Drawing for the job (mm, zero at the part's lowest x, y, z). A direction names the side the tool comes from. Give positions to 0.01 mm unless a question says otherwise; leave off trailing zeros. Loops run counter-clockwise (first coordinate to the right, second up) from the corner with the lowest first, then second, coordinate; pieces in that order, holes last. Notation, with made-up numbers: (40, -36) -> (92, -36) arc R23 ccw to (92, -20) -> close; hole circle Ø7 at (-5.5, -22.5). An arc over 180 degrees is marked (long way). Answer in a Markdown table with one row per item. Add a question column.
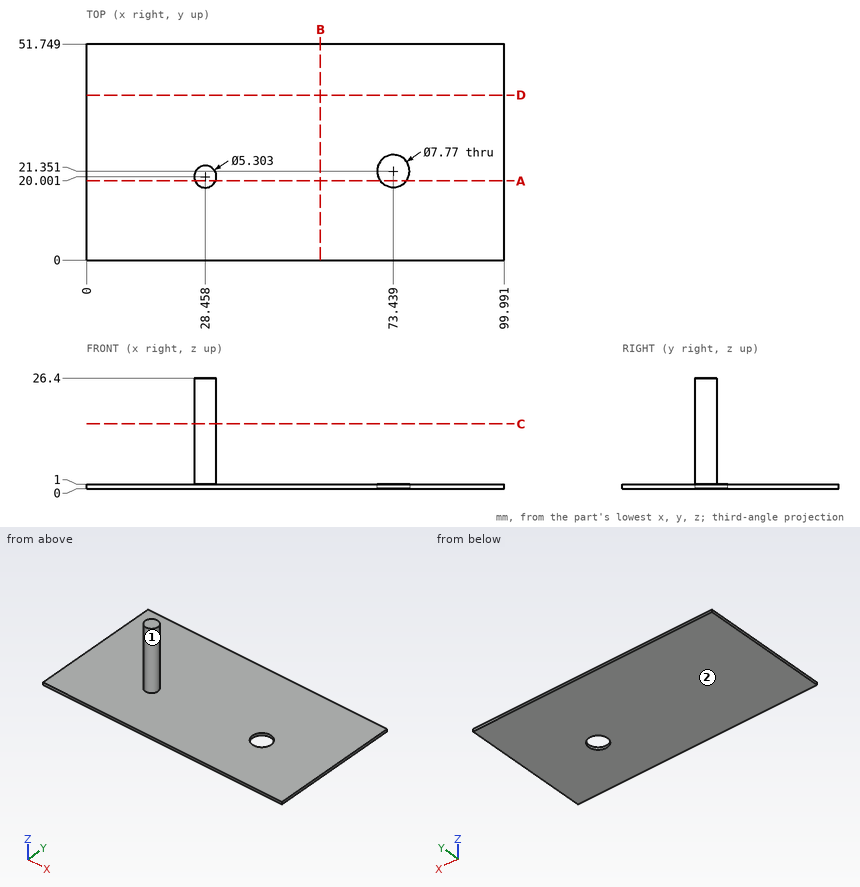
(1) Wall check: line 1 along Z through (x, y) = (18.5, 49); line 2 along X through (y, z) = (18, 12.75) (1 decimal). Give the ranges that are in metal, low to high. Write a range as from..to.
(2) Saw through at D-D, the plane y = 39.5. List the corners of the cut face in (x, z).
(3) Flat gauge pins, fed straight in: pin 1 Ø15.5 at (x, y) = (75, 25) entering from +Z; pin 2 Ø3 at (y, z) = (21, 3) entering from +X. Where does each tip first touch, or does it go through?
(4) Saw through at B-B, the plane x = 56. List the corners of the cut face in (y, z).
(5) 3-axis set-ups, long thin cutter, end or side, ignore diameter. For the marked faces 1 and 2: which of +Z, -Z, +X, -X, +Y, -Y reach the whole face in a straight line?
(6) Saw through at C-C, the plane z = 15.5. List the corners of the cut face in (x, y).
(7) Saw through at A-A, the plane y = 19. List the corners of the cut face in (x, z).
Worked answers:
| question | item | result |
|---|---|---|
| 1 | line 1 | 0..1 |
| 1 | line 2 | 26.7..30.2 |
| 2 | outline | (0, 0) -> (99.99, 0) -> (99.99, 1) -> (0, 1) -> close |
| 3 | pin 1 | z = 1 |
| 3 | pin 2 | x = 31.11 |
| 4 | outline | (0, 0) -> (51.75, 0) -> (51.75, 1) -> (0, 1) -> close |
| 5 | face 1 | +Z |
| 5 | face 2 | -Z, +X, -X, +Y, -Y |
| 6 | outline | circle Ø5.3 at (28.46, 20) |
| 7 | outline | (0, 0) -> (70.35, 0) -> (70.35, 1) -> (30.91, 1) -> (30.91, 26.4) -> (26, 26.4) -> (26, 1) -> (0, 1) -> close; (76.53, 0) -> (99.99, 0) -> (99.99, 1) -> (76.53, 1) -> close |
